```python
from build123d import *

# Parameters (mm, degrees)
ESBO_O1_W                = 555
ESBO_O1_H                = 200
RESSALTO_EXTRUS_O1_DEPTH = 3
ESBO_O2_W                = 3.5
ESBO_O2_H                = 31
ESBO_O2_W_2              = 31
ESBO_O2_H_2              = 3.5
CORTE_EXTRUS_O1_DEPTH    = 295.983474113
CORTE_EXTRUS_O2_DEPTH    = 295.983474113


with BuildPart() as part:
    # Esboço1 → Ressalto-extrusão1 (new body)
    with BuildSketch(Plane.XY):
        Rectangle(ESBO_O1_W, ESBO_O1_H)
    extrude(amount=RESSALTO_EXTRUS_O1_DEPTH)

    # Esboço2 → Corte-extrusão1 (cut, through all)
    with BuildSketch(Plane.XY.offset(3)):
        with Locations((237.25, 0)):
            Rectangle(ESBO_O2_W, ESBO_O2_H)
        with Locations((-153.75, 0)):
            Rectangle(ESBO_O2_W, ESBO_O2_H)
        with Locations((-237.25, 0)):
            Rectangle(ESBO_O2_W, ESBO_O2_H)
        with Locations((-195.5, 41.75)):
            Rectangle(ESBO_O2_W_2, ESBO_O2_H_2)
        with Locations((-195.5, -41.75)):
            Rectangle(ESBO_O2_W_2, ESBO_O2_H_2)
        with Locations((153.75, 0)):
            Rectangle(ESBO_O2_W, ESBO_O2_H)
        with Locations((195.5, -41.75)):
            Rectangle(ESBO_O2_W_2, ESBO_O2_H_2)
        with Locations((195.5, 41.75)):
            Rectangle(ESBO_O2_W_2, ESBO_O2_H_2)
    extrude(amount=-CORTE_EXTRUS_O1_DEPTH, mode=Mode.SUBTRACT)

    # Esboço3 → Corte-extrusão2 (cut, through all)
    with BuildSketch(Plane.XY.offset(3)):
        Polygon((0, 100), (0, 50), (15, 50), (15, -50), (0, -50), (0, -100), (277.5, -100), (277.5, 100), align=None)
    extrude(amount=-CORTE_EXTRUS_O2_DEPTH, mode=Mode.SUBTRACT)


solid = part.part
```
Source: CAD feature listing. Evaluate the final solid. Frame: model axes, mm. Round coordinates to 2 decimals unless told otherwise and drop trailing zeros. Loops run counter-clockwise (first coordinate to the right, second up) from the corner with the lowest first, then second, coordinate; pieces in that order, holes last.
(1) Section query C-C (y = -58). Output: boundary loops of the cut face in (x, z).
From the geometry:
outline: (-277.5, 0) - (0, 0) - (0, 3) - (-277.5, 3) - close
(2) Section query B-B (x = -184.5). Output: boundary loops of the cut face in (y, z), and give its area (3 significant figures).
From the geometry:
outline: (-100, 0) - (-43.5, 0) - (-43.5, 3) - (-100, 3) - close; (-40, 0) - (40, 0) - (40, 3) - (-40, 3) - close; (43.5, 0) - (100, 0) - (100, 3) - (43.5, 3) - close
area: 579 mm2
(3) Material intervals for probe 1 along Y at (x, z) = (-181, 1.4); probe 2 along X at (y, z) = (-1, 1.6); probe 3 along X at (y, z) = (41, 0.2), sorted ascending.
From the geometry:
probe 1: y = -100 to -43.5, -40 to 40, 43.5 to 100
probe 2: x = -277.5 to -239, -235.5 to -155.5, -152 to 15
probe 3: x = -277.5 to -211, -180 to 15
(4) Contact query for flat-ended pins moving along their axis: pin 1 Ø1.5 at (y, z) = (64, 1) entering from +X; pin 2 Ø1.5 at (x, z) = (9.5, 1) entering from -Y. Output: stop coordinate, or through.
From the geometry:
pin 1: stops at x = 0
pin 2: stops at y = -50
(5) Section query A-A (z = 1). Output: boundary loops of the cut face in (x, y), and give its area (3 significant figures).
From the geometry:
outline: (-277.5, -100) - (0, -100) - (0, -50) - (15, -50) - (15, 50) - (0, 50) - (0, 100) - (-277.5, 100) - close; hole (-239, -15.5) - (-235.5, -15.5) - (-235.5, 15.5) - (-239, 15.5) - close; hole (-211, -43.5) - (-180, -43.5) - (-180, -40) - (-211, -40) - close; hole (-211, 40) - (-180, 40) - (-180, 43.5) - (-211, 43.5) - close; hole (-155.5, -15.5) - (-152, -15.5) - (-152, 15.5) - (-155.5, 15.5) - close
area: 56,600 mm2
